Can you work these out from the model? Positions are in its coordinate system, mm. A direction names the side the tool comes from. Round coordinates to 2 decimals unless told otherwise and drop trailing zeros. Write each loop counter-clockwise with the first axis right and the second up, starting at its lowest first coordinate (ties: lowest second). Pieces come first, ordered by that corner, then holes. Notation, with made-up numbers: (79, 15) - (133, 15) arc R26 ccw to (133, 43) - close; hole circle Ø3 at (-9.5, -3.5). An arc over 180 degrees is marked (long way). One line per item, written item: value. Start each with the question number.
(1) I want a section at A-A on z = 7.5. List the corners of the cut face in (x, y) for me, plus the area to 3 significant figures.
(2) If I drill on L1, parallel to Z at x = 3, y = 76.5; L2, parallel to Y at x = -2, z = 4.75; L3, parallel to Y at x = 67, z = 2.5, over which ranges is the centre line in solid material (lowest first)? Write a range as from..to.
(3) I'm going to push flat-ended pins straight in: pin 1 Ø1.9 at (x, y) = (40.94, 41.54) entering from +Z; pin 2 Ø1.5 at (x, z) = (16.5, 3) entering from +Y; pin 3 Ø5 at (x, z) = (5, 6.5) entering from +Y; pin 4 Ø1.5 at (y, z) = (44.5, 1.5) entering from +X. Where does each tip first touch, or does it pass through?
(4) I want a section at C-C on x = 32.5. List the corners of the cut face in (y, z) for me, plus the area to 3 significant figures.
(5) I want a section at B-B on y = 28. List the corners of the cut face in (x, z) for me (3 decimals).
(6) On a 3-axis mill with a long thin cutter (end or side, diameter ignored), from which of +Z, -Z, +X, -X, +Y, -Y can I reach the whole of each face in a straight line? I mean faces 1 (the face through (39.6, 47.6, 9)), 2 (the face through (77.486, 0.373, 4.93)). Say none if no direction works.
(7) Thinking about a two-plate mould opening in Y: for faces 3 (the face through (34.46, 42.21, 5.06)), 4 (the face through (36.4, 42.5, 0)), 5 (the face through (32.5, 42.7, 4.9)), which applies, +Y half, -Y half, draft (parallel to the pull), parting line (faces both ways), or undercut?
(8) I want a section at D-D on x = 22. List the corners of the cut face in (y, z) for me.
from build123d import *

# Parameters (mm, degrees)
SKETCH_2_R          = 1.6
EXTRUDE_1_DEPTH     = 10
SKETCH_3_W          = 8
SKETCH_3_H          = 8
CUT_EXTRUDE_1_DEPTH = 140.947387002
SKETCH_4_R          = 1.6
SKETCH_4_R_2        = 3
CUT_EXTRUDE_2_DEPTH = 10


with BuildPart() as part:
    # ｽｹｯﾁ2 → ﾎﾞｽ - 押し出し1 (new body)
    with BuildSketch(Plane.XY):
        Polygon((83.071643169, 8.195972832), (-3.936021884, 91.354077293), (-10.845357286, 84.124894469), (77.150331852, 0.022479987), (84.059667254, 7.25166281), align=None)
        with Locations((-3.776098173, 84.28481818)):
            Circle(SKETCH_2_R, mode=Mode.SUBTRACT)
        with Locations((76.990408141, 7.0917391)):
            Circle(SKETCH_2_R, mode=Mode.SUBTRACT)
    extrude(amount=EXTRUDE_1_DEPTH)

    # ｽｹｯﾁ3 → ｶｯﾄ - 押し出し1 (cut, through all)
    with BuildSketch(Plane(origin=(40.308371471, -38.524970914, 0), x_dir=(0, 0, -1), z_dir=(0.7229182823698357, -0.690933540230496, 0))):
        with Locations((-5, 58.32200311)):
            Rectangle(SKETCH_3_W, SKETCH_3_H)
    extrude(amount=-CUT_EXTRUDE_1_DEPTH, mode=Mode.SUBTRACT)

    # ｽｹｯﾁ4 → ｶｯﾄ - 押し出し2 (cut)
    with BuildSketch(Plane.XY.offset(10)):
        with Locations((40.944664678, 41.542677398)):
            Circle(SKETCH_4_R)
        with Locations((32.26964529, 49.833879881)):
            Circle(SKETCH_4_R)
        with Locations((36.607154984, 45.68827864)):
            Circle(SKETCH_4_R_2)
    extrude(amount=-CUT_EXTRUDE_2_DEPTH, mode=Mode.SUBTRACT)


solid = part.part
Established:
1. outline: (-10.85, 84.12) - (77.15, 0.02) - (77.84, 0.75) - (-10.15, 84.85) - close; (-4.63, 90.63) - (83.37, 6.53) - (84.06, 7.25) - (-3.94, 91.35) - close
1. area: 243 mm2
2. L1: 0..1, 9..10
2. L2: 75.67..77.05, 88.12..89.5
2. L3: 9.72..11.11, 22.17..23.56
3. pin 1: through
3. pin 2: y = 72.54
3. pin 3: y = 85.2
3. pin 4: x = 45.87
4. outline: (42.7, 0) - (48.25, 0) - (48.25, 1) - (44.08, 1) - (44.08, 9) - (48.25, 9) - (48.25, 10) - (42.7, 10) - close; (51.42, 0) - (56.53, 0) - (56.53, 10) - (51.42, 10) - (51.42, 9) - (55.15, 9) - (55.15, 1) - (51.42, 1) - close
4. area: 43.5 mm2
5. outline: (47.878, 0) - (62.351, 0) - (62.351, 10) - (47.878, 10) - close; hole (49.325, 1) - (60.904, 1) - (60.904, 9) - (49.325, 9) - close
6. face 1: none
6. face 2: +Z, -Z, +X, -Y
7. face 3: undercut
7. face 4: draft
7. face 5: -Y half
8. outline: (52.73, 0) - (66.57, 0) - (66.57, 10) - (52.73, 10) - close; hole (54.12, 1) - (65.18, 1) - (65.18, 9) - (54.12, 9) - close
